Check sheet for the modelled part. Datum: model origin and axes. Units: mm. Face numbers are marked on the shaded views. A direction names the side the tool comes from. Coordinates: 2 decimals unless noted, no trailing zeros. Write each loop counter-clockwise with the first axis right and the second up, starting at its lowest first coordinate (ties: lowest second). Pieces come first, ordered by that corner, then holes. Notation, with made-up numbers: M -35.75,8 L -29.75,8 A11 ccw -29.75,15 Z; hole C 22.5,54.25 d10. An arc over 180 degrees is marked long. Answer as CSV lines item,"result". Start each with the question number.
1) Draft check along Y on the marked faces 1, 2 and 3. Enter one of: +Y half, -Y half, draft (parallel to the pull), parting line (faces both ways), or undercut.
2) Section check C-C (y = -14.25). Record the cut outline in (x, z), and give its area (3 significant figures).
3) Material ranges on L1, parallel to X at y = -13.75, z = -18.25; L2, parallel to Y at x = 17, z = -18.25; L3, parallel to X at y = -1.75, z = -7.5, recorded low to high. Write a range as [from, to].
4) Go/stop test with flat-tipped pins: pin 1 Ø9.5 at (y, z) = (-4.5, -9) entering from +X; pin 2 Ø10 at (x, z) = (13.5, -8) entering from +Y; pin 3 Ø1 at (y, z) = (-14, -10) entering from +X. Record where each tip stops, or that it passes through.
5) Access from +Z, -Z, +X, -X, +Y, -Y to the whole of each face (thin tool, end or side, straight path). Record for the marked faces 4 and 5.
6) Section check A-A (x = 25). Record the cut outline in (y, z).
7) Section check B-B (z = -4.5). Record the cut outline in (x, y), and give its area (3 significant figures).
8) Section check D-D (z = -11.5). Record the cut outline in (x, y).
from build123d import *

# Parameters (mm, degrees)
SKETCH3_W                = 20
SKETCH3_H                = 12
BOSS_EXTRUDE3_DEPTH      = 2
BOSS_EXTRUDE5_DEPTH      = 32
BOSS_EXTRUDE5_DEPTH_BACK = 2
SKETCH4_W                = 20
SKETCH4_H                = 5
CUT_EXTRUDE1_DEPTH       = 30
SKETCH7_W                = 20
SKETCH7_H                = 2
CUT_EXTRUDE2_DEPTH       = 43.95346319


with BuildPart() as part:
    # Sketch3 → Boss-Extrude3 (new body)
    with BuildSketch(Plane(origin=(0, 0, 0), x_dir=(0, 0, -1), z_dir=(1, 0, 0))):
        with Locations((10, -6)):
            Rectangle(SKETCH3_W, SKETCH3_H)
    extrude(amount=BOSS_EXTRUDE3_DEPTH)

    # Sketch4 → Boss-Extrude5 (add, two sides: drawn at the far end of the back side and taken through both)
    with BuildSketch(Plane(origin=(2, 0, 0), x_dir=(0, 0, -1), z_dir=(1, 0, 0)).offset(-BOSS_EXTRUDE5_DEPTH_BACK)):
        with Locations((10, -14.5)):
            Rectangle(SKETCH4_W, SKETCH4_H)
    extrude(amount=BOSS_EXTRUDE5_DEPTH + BOSS_EXTRUDE5_DEPTH_BACK)

    # Sketch6 → Cut-Extrude1 (cut)
    with BuildSketch(Plane(origin=(34, 0, 0), x_dir=(0, 0, -1), z_dir=(1, 0, 0))):
        Polygon((5, -15.5), (15, -15.5), (12.5, -12), (7.5, -12), align=None)
    extrude(amount=-CUT_EXTRUDE1_DEPTH, mode=Mode.SUBTRACT)

    # Sketch7 → Cut-Extrude2 (cut, through all)
    with BuildSketch(Plane(origin=(0, 0, -20), x_dir=(-1, 0, 0), z_dir=(0, 0, -1))):
        with Locations((-20, -14.5)):
            Rectangle(SKETCH7_W, SKETCH7_H)
    extrude(amount=-CUT_EXTRUDE2_DEPTH, mode=Mode.SUBTRACT)


solid = part.part
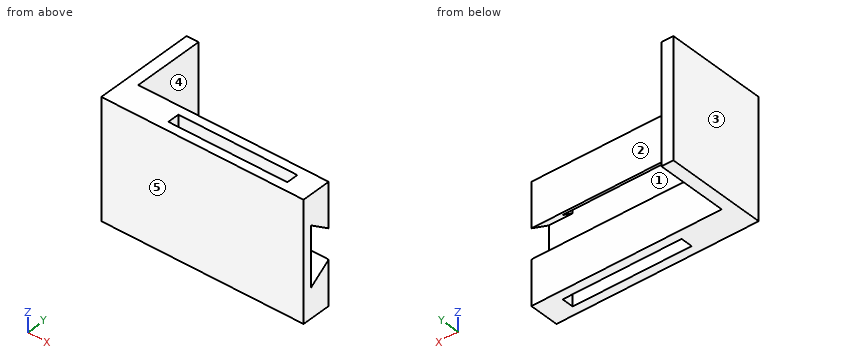
Results found:
1,face 1,"undercut"
1,face 2,"+Y half"
1,face 3,"draft"
2,outline,"M 0,-20 L 10,-20 L 10,-14.11 L 4,-14.11 L 4,-5.89 L 10,-5.89 L 10,0 L 0,0 Z; M 30,-20 L 34,-20 L 34,-14.11 L 30,-14.11 Z; M 30,-5.89 L 34,-5.89 L 34,0 L 30,0 Z"
2,area,"198 mm2"
3,L1,"x = [0, 10], [30, 34]"
3,L2,"y = [-17, -15.5], [-13.5, -12]"
3,L3,"x = [0, 2]"
4,pin 1,"stops at x = 2"
4,pin 2,"stops at y = -12"
4,pin 3,"stops at x = 4"
5,face 4,"+Z, -Z, +X, +Y"
5,face 5,"+Z, -Z, +X, -X, -Y"
6,outline,"M -17,-20 L -15.5,-20 L -15.5,0 L -17,0 Z; M -13.5,-20 L -12,-20 L -12,-12.5 L -13.5,-13.57 Z; M -13.5,-6.43 L -12,-7.5 L -12,0 L -13.5,0 Z"
7,outline,"M 0,-17 L 34,-17 L 34,-12 L 2,-12 L 2,0 L 0,0 Z; hole M 10,-15.5 L 30,-15.5 L 30,-13.5 L 10,-13.5 Z"
7,area,"154 mm2"
8,outline,"M 0,-17 L 34,-17 L 34,-15.5 L 4,-15.5 L 4,-12 L 2,-12 L 2,0 L 0,0 Z"
